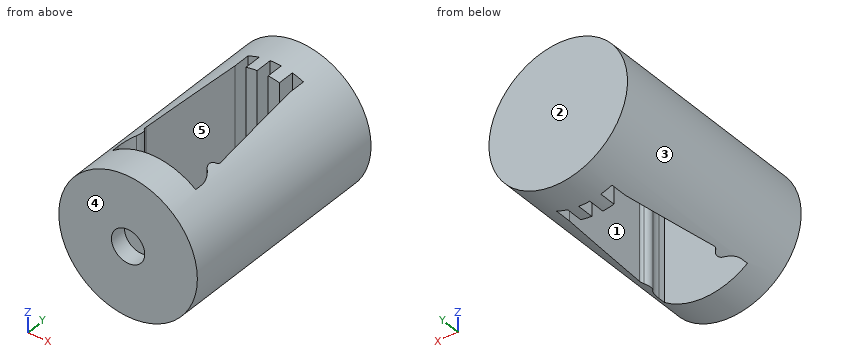
from build123d import *

# Parameters (mm, degrees)
SKETCH2_R               = 12.5
BOSS_EXTRUDE1_DEPTH     = 20
CUT_EXTRUDE1_DEPTH      = 13.5
CUT_EXTRUDE1_DEPTH_BACK = 13.5
SKETCH4_R               = 3
CUT_EXTRUDE2_DEPTH      = 3


with BuildPart() as part:
    # Sketch2 → Boss-Extrude1 (new body, symmetric)
    with BuildSketch(Plane(origin=(0, 0, 0), x_dir=(1, 0, 0), z_dir=(0, 1, 0))):
        Circle(SKETCH2_R)
    extrude(amount=BOSS_EXTRUDE1_DEPTH, both=True)

    # Sketch3 → Cut-Extrude1 (cut, two sides)
    with BuildSketch(Plane.XY) as cut_extrude1_sk:
        with BuildLine():
            Line((-7.5, -14), (7.5, -14))
            Line((7.5, -14), (7.5, -12.75))
            ThreePointArc((7.5, -12.75), (7.203207399, -11.211161096), (6.35540622, -9.893077571))
            ThreePointArc((6.35540622, -9.893077571), (5.999449038, -8.930951878), (6.455951755, -8.012258985))
            ThreePointArc((6.455951755, -8.012258985), (6.691617305, -7.687574573), (6.749863955, -7.290629305))
            Line((6.749863955, -7.290629305), (5, 11))
            Line((5, 11), (5, 14))
            Line((5, 14), (3, 14))
            Line((3, 14), (3, 11))
            Line((3, 11), (1, 11))
            Line((1, 11), (1, 14))
            Line((1, 14), (-1, 14))
            Line((-1, 14), (-1, 11))
            Line((-1, 11), (-3, 11))
            Line((-3, 11), (-3, 14))
            Line((-3, 14), (-5, 14))
            Line((-5, 14), (-5, 11))
            Line((-5, 11), (-6.749863955, -7.290629305))
            ThreePointArc((-6.749863955, -7.290629305), (-6.691617305, -7.687574573), (-6.455951755, -8.012258985))
            ThreePointArc((-6.455951755, -8.012258985), (-5.999449038, -8.930951878), (-6.35540622, -9.893077571))
            ThreePointArc((-6.35540622, -9.893077571), (-7.203207399, -11.211161096), (-7.5, -12.75))
            Line((-7.5, -12.75), (-7.5, -14))
        make_face()
    extrude(amount=CUT_EXTRUDE1_DEPTH, mode=Mode.SUBTRACT)
    extrude(cut_extrude1_sk.sketch, amount=-CUT_EXTRUDE1_DEPTH_BACK, mode=Mode.SUBTRACT)

    # Sketch4 → Cut-Extrude2 (cut)
    with BuildSketch(Plane(origin=(0, -20, 0), x_dir=(-1, 0, 0), z_dir=(0, -1, 0))):
        Circle(SKETCH4_R)
    extrude(amount=-CUT_EXTRUDE2_DEPTH, mode=Mode.SUBTRACT)


solid = part.part
CAD build for the part. Positions are in the model's coordinates, mm. Face numbers are marked on the shaded views. A direction names the side the tool comes from. Round coordinates to 2 decimals unless told otherwise and drop trailing zeros. Loops run counter-clockwise (first coordinate to the right, second up) from the corner with the lowest first, then second, coordinate; pieces in that order, holes last.
(1) Wall check: line 1 along X through (y, z) = (-18, 0); line 2 along Y through (x, z) = (-4, 11); line 3 along Y through (x, z) = (1.25, -2.25). Give the ranges that are in metal, low to high.
(2) Two-plate mould, pull along X, no slides. Class the marked faces 3, 4 and 5: +X half, -X half, draft (parallel to the pull), parting line (faces both ways), or undercut.
(3) Drop flat-ended pins along their axis: pin 1 (12 mm diameter, centred on y = -7, z = 8, fed in from -X); pin 2 (2.5 mm diameter, centred on y = 12.5, z = -1.5, fed in from +X); pin 3 (3 mm diameter, centred on x = -5.5, y = -3, fed in from +Z). Give the stop position or say it passes through.
(4) Cut at A-A (x = 0). Give the cut face in (y, z), plus the area to 3 significant figures.
(5) Cut at D-D (x = -5.5). Give the cut face in (y, z), plus the area to 3 significant figures.
(6) Cut at C-C (y = -15). Give the cut face in (x, z), plus the area to 3 significant figures.
(7) Which spindle directions (+Z, -Z, +X, -X, +Y, -Y) get a long thin tool onto all of the face, cutting with end or side? Do the marked faces 1 and 2. Say none if no direction does.
Findings below:
1. line 1: x = -12.5 to -3, 3 to 12.5
1. line 2: y = -20 to -14, 14 to 20
1. line 3: y = -17 to -14, 11 to 20
2. face 3: parting line
2. face 4: draft
2. face 5: undercut
3. pin 1: stops at x = -12.34
3. pin 2: stops at x = 12.5
3. pin 3: stops at z = 10.85
4. outline: (-20, -12.5) - (-14, -12.5) - (-14, 12.5) - (-20, 12.5) - (-20, 3) - (-17, 3) - (-17, -3) - (-20, -3) - close; (14, -12.5) - (20, -12.5) - (20, 12.5) - (14, 12.5) - close
4. area: 282 mm2
5. outline: (-20, -11.22) - (-14, -11.22) - (-14, 11.22) - (-20, 11.22) - close; (5.77, -11.22) - (20, -11.22) - (20, 11.22) - (5.77, 11.22) - close
5. area: 454 mm2
6. outline: circle Ø25 at (0, 0)
6. area: 491 mm2
7. face 1: +Z, -Z
7. face 2: +Z, -Z, +X, -X, +Y
